```python
from build123d import *

# Parameters (mm, degrees)
CROQUIS1_W                              = 145
CROQUIS1_H                              = 105
SALIENTE_EXTRUIR1_DEPTH                 = 39
TALADRO1_D                              = 14
SIMETR_A2_COPY_1_D                      = 14
TALADRO_DE_MARGEN_PARA_M1_61_AT_2_COUNT = 2
TALADRO_DE_MARGEN_PARA_M1_61_AT_2_PITCH = 15
TALADRO_DE_MARGEN_PARA_M1_61_AT_3_COUNT = 2
TALADRO_DE_MARGEN_PARA_M1_61_AT_3_PITCH = 30
TALADRO_DE_MARGEN_PARA_M1_62_AT_2_COUNT = 2
TALADRO_DE_MARGEN_PARA_M1_62_AT_2_PITCH = 40.311288741
TALADRO_DE_MARGEN_PARA_M1_62_AT_3_COUNT = 2
TALADRO_DE_MARGEN_PARA_M1_62_AT_3_PITCH = 40.311288741
CORTAR_EXTRUIR1_DEPTH                   = 3
SIMETR_A6_COPY_1_DEPTH                  = 3


with BuildPart() as part:
    # Croquis1 → Saliente-Extruir1 (new body)
    with BuildSketch(Plane.XY):
        Rectangle(CROQUIS1_W, CROQUIS1_H)
    extrude(amount=SALIENTE_EXTRUIR1_DEPTH)

    # Taladro1 (through all)
    with Locations(Plane.XY.offset(39)):
        with Locations((-57.5, 38.5)):
            taladro1 = Hole(TALADRO1_D / 2)

    # Simetría1: Taladro1 across plane
    add(taladro1.mirror(Plane.ZX), mode=Mode.SUBTRACT)

    # Simetría2: Taladro1 across plane
    add(taladro1.mirror(Plane(origin=(0, 0, 0), x_dir=(0, 0, 1), z_dir=(1, 0, 0))), mode=Mode.SUBTRACT)

    # Simetría2 copy 1 (through all)
    with Locations(Plane(origin=(0, 0, 39), x_dir=(-1, 0, 0), z_dir=(0, 0, 1))):
        with Locations((-57.5, 38.5)):
            Hole(SIMETR_A2_COPY_1_D / 2)

    # Croquis7 → Taladro de margen para M1.61 (revolve, cut)
    with BuildSketch(Plane(origin=(0, 40, 39), x_dir=(0, -1, 0), z_dir=(1, 0, 0))):
        Polygon((0, 0), (0, 28.004303095), (5, 25), (5, 0), align=None)
    taladro_de_margen_para_m1_61 = revolve(axis=Axis((0, 40, 45.35), (0, 0, -1)), mode=Mode.SUBTRACT)

    # Taladro de margen para M1.61 at 2: Taladro de margen para M1.61 ×2
    with Locations(*[(0, -i * TALADRO_DE_MARGEN_PARA_M1_61_AT_2_PITCH, 0) for i in range(1, TALADRO_DE_MARGEN_PARA_M1_61_AT_2_COUNT)]):
        add(taladro_de_margen_para_m1_61, mode=Mode.SUBTRACT)

    # Taladro de margen para M1.61 at 3: Taladro de margen para M1.61 ×2
    with Locations(*[(0, -i * TALADRO_DE_MARGEN_PARA_M1_61_AT_3_PITCH, 0) for i in range(1, TALADRO_DE_MARGEN_PARA_M1_61_AT_3_COUNT)]):
        add(taladro_de_margen_para_m1_61, mode=Mode.SUBTRACT)

    # Simetría3: Taladro de margen para M1.61 across plane
    add(taladro_de_margen_para_m1_61.mirror(Plane.ZX), mode=Mode.SUBTRACT)

    # Simetría3 copy 1 sketch → Simetría3 copy 1 (revolve, cut)
    with BuildSketch(Plane(origin=(0, -25, 39), x_dir=(0, 1, 0), z_dir=(1, 0, 0))):
        Polygon((0, 0), (0, -28.004303095), (5, -25), (5, 0), align=None)
    revolve(axis=Axis((0, -25, 45.35), (0, 0, 1)), mode=Mode.SUBTRACT)

    # Simetría3 copy 2 sketch → Simetría3 copy 2 (revolve, cut)
    with BuildSketch(Plane(origin=(0, -10, 39), x_dir=(0, 1, 0), z_dir=(1, 0, 0))):
        Polygon((0, 0), (0, -28.004303095), (5, -25), (5, 0), align=None)
    revolve(axis=Axis((0, -10, 45.35), (0, 0, 1)), mode=Mode.SUBTRACT)

    # Croquis9 → Taladro de margen para M1.62 (revolve, cut)
    with BuildSketch(Plane(origin=(-57.5, 0, 39), x_dir=(0, -1, 0), z_dir=(1, 0, 0))):
        Polygon((0, 0), (0, 21.605163714), (6, 18), (6, 0), align=None)
    taladro_de_margen_para_m1_62 = revolve(axis=Axis((-57.5, 0, 45.35), (0, 0, -1)), mode=Mode.SUBTRACT)

    # Taladro de margen para M1.62 at 2: Taladro de margen para M1.62 ×2
    with Locations(*[Vector(0.868243142, 0.496138938, 0) * (i * TALADRO_DE_MARGEN_PARA_M1_62_AT_2_PITCH) for i in range(1, TALADRO_DE_MARGEN_PARA_M1_62_AT_2_COUNT)]):
        add(taladro_de_margen_para_m1_62, mode=Mode.SUBTRACT)

    # Taladro de margen para M1.62 at 3: Taladro de margen para M1.62 ×2
    with Locations(*[Vector(0.868243142, -0.496138938, 0) * (i * TALADRO_DE_MARGEN_PARA_M1_62_AT_3_PITCH) for i in range(1, TALADRO_DE_MARGEN_PARA_M1_62_AT_3_COUNT)]):
        add(taladro_de_margen_para_m1_62, mode=Mode.SUBTRACT)

    # Simetría4: Taladro de margen para M1.62 across plane
    add(taladro_de_margen_para_m1_62.mirror(Plane(origin=(0, 0, 0), x_dir=(0, 0, 1), z_dir=(1, 0, 0))), mode=Mode.SUBTRACT)

    # Simetría4 copy 1 sketch → Simetría4 copy 1 (revolve, cut)
    with BuildSketch(Plane(origin=(22.5, 20, 39), x_dir=(0, -1, 0), z_dir=(-1, 0, 0))):
        Polygon((0, 0), (0, -21.605163714), (6, -18), (6, 0), align=None)
    revolve(axis=Axis((22.5, 20, 45.35), (0, 0, 1)), mode=Mode.SUBTRACT)

    # Simetría4 copy 2 sketch → Simetría4 copy 2 (revolve, cut)
    with BuildSketch(Plane(origin=(22.5, -20, 39), x_dir=(0, -1, 0), z_dir=(-1, 0, 0))):
        Polygon((0, 0), (0, -21.605163714), (6, -18), (6, 0), align=None)
    revolve(axis=Axis((22.5, -20, 45.35), (0, 0, 1)), mode=Mode.SUBTRACT)

    # Croquis10 → Cortar-Extruir1 (cut)
    with BuildSketch(Plane.XY.offset(39)):
        with BuildLine():
            Line((-37.5, 52.5), (-37.5, 26.5))
            ThreePointArc((-37.5, 26.5), (-40.428932188, 19.428932188), (-47.5, 16.5))
            Line((-47.5, 16.5), (-72.5, 16.5))
            Line((-72.5, 16.5), (-72.5, 18.5))
            Line((-72.5, 18.5), (-49.5, 18.5))
            ThreePointArc((-49.5, 18.5), (-42.428932188, 21.428932188), (-39.5, 28.5))
            Line((-39.5, 28.5), (-39.5, 52.5))
            Line((-39.5, 52.5), (-37.5, 52.5))
        make_face()
    cortar_extruir1 = extrude(amount=-CORTAR_EXTRUIR1_DEPTH, mode=Mode.SUBTRACT)

    # Simetría5: Cortar-Extruir1 across plane
    add(cortar_extruir1.mirror(Plane.ZX), mode=Mode.SUBTRACT)

    # Simetría6: Cortar-Extruir1 across plane
    add(cortar_extruir1.mirror(Plane(origin=(0, 0, 0), x_dir=(0, 0, 1), z_dir=(1, 0, 0))), mode=Mode.SUBTRACT)

    # Simetría6 copy 1 sketch → Simetría6 copy 1 (cut)
    with BuildSketch(Plane(origin=(0, 0, 39), x_dir=(-1, 0, 0), z_dir=(0, 0, 1))):
        with BuildLine():
            Line((-37.5, 52.5), (-37.5, 26.5))
            ThreePointArc((-37.5, 26.5), (-40.428932188, 19.428932188), (-47.5, 16.5))
            Line((-47.5, 16.5), (-72.5, 16.5))
            Line((-72.5, 16.5), (-72.5, 18.5))
            Line((-72.5, 18.5), (-49.5, 18.5))
            ThreePointArc((-49.5, 18.5), (-42.428932188, 21.428932188), (-39.5, 28.5))
            Line((-39.5, 28.5), (-39.5, 52.5))
            Line((-39.5, 52.5), (-37.5, 52.5))
        make_face()
    extrude(amount=-SIMETR_A6_COPY_1_DEPTH, mode=Mode.SUBTRACT)


solid = part.part
```
Geometry: final body of the model. Coordinates: model frame, mm. A direction names the side the tool comes from. Give positions to 0.01 mm unless a question says otherwise; leave off trailing zeros. Write each loop counter-clockwise with the first axis right and the second up, starting at its lowest first coordinate (ties: lowest second). Pieces come first, ordered by that corner, then holes.
1. Reachability of faces 5 (the flat face through (39.5, -40, 38)), 6 (the flat face through (60, 16.5, 38)), 7 (the cylindrical face through (0, -45, 27)), 8 (the flat face through (-1, -52.5, 19)) from +Z, -Z, +X, -X, +Y, -Y: full face, straight path, thin tool, end or side. Return the list, or none.
2. Draft query along Y for faces 1 (the conical face through (0.53, 10.69, 11.52)), 2 (the flat face through (37.5, 40, 38)), 3 (the flat face through (-1, 52.5, 19)), 4 (the cylindrical face through (40.35, -19.51, 37.52)). Return one class per face: released by +Y, released by -Y, zero draft, split by the parting line, or undercut.
3. Line query: probe 1 along Y at (x, z) = (58, 29.5); probe 2 along X at (y, z) = (0, 34.75); probe 3 along Y at (x, z) = (57.5, 8). Output: solid intervals per line, ascending.
4. Section query B-B, the plane y = 38.5. Count the separate pieces of the cut face and the enclosed holes in it, then the cut area to 3 significant figures.
5. Section query A-A, the plane z = 3. Return loops of the section in (x, y).
Computed:
1. face 5: +Z, -Y
1. face 6: +Z, +X
1. face 7: +Z
1. face 8: +Z, -Z, +X, -X, -Y
2. face 1: undercut
2. face 2: zero draft
2. face 3: released by +Y
2. face 4: undercut
3. probe 1: y = -52.5 to -45.48, -31.52 to -5.98, 5.98 to 31.52, 45.48 to 52.5
3. probe 2: x = -72.5 to -63.5, -51.5 to 51.5, 63.5 to 72.5
3. probe 3: y = -52.5 to -45.5, -31.5 to 31.5, 45.5 to 52.5
4. separate pieces: 3
4. enclosed holes: 0
4. area: 4,300 mm2
5. outline: (-72.5, -52.5) - (72.5, -52.5) - (72.5, 52.5) - (-72.5, 52.5) - close; hole circle Ø14 at (-57.5, -38.5); hole circle Ø14 at (-57.5, 38.5); hole circle Ø14 at (57.5, -38.5); hole circle Ø14 at (57.5, 38.5)
